from build123d import *

# Parameters (mm, degrees)
BOSS_EXTRUDE1_DEPTH = 3.175
CAVITY1_DEPTH       = 3.175


# Read off the part's stored shape, not the designer's step: Cavity1
with BuildPart() as part:
    # Sketch1 → Boss-Extrude1 (new body)
    with BuildSketch(Plane.XY):
        with BuildLine():
            Line((-9.017779189, 0), (0, 0))
            Line((0, 0), (0, 1.852083291))
            ThreePointArc((0, 1.852083291), (-2.38125, 4.233333291), (0, 6.614583291))
            Line((0, 6.614583291), (0, 20.902083291))
            ThreePointArc((0, 20.902083291), (-2.38125, 23.283333291), (0, 25.664583291))
            Line((0, 25.664583291), (0, 27.516666667))
            Line((0, 27.516666667), (-7.878035599, 27.516666667))
            ThreePointArc((-7.878035599, 27.516666667), (-12.19254052, 25.825802562), (-14.209331582, 21.653689435))
            Line((-14.209331582, 21.653689435), (-15.349075172, 6.837022768))
            ThreePointArc((-15.349075172, 6.837022768), (-13.676915084, 2.035495079), (-9.017779189, 0))
        make_face()
        with BuildLine():
            Line((0, 1.852083291), (0, 0))
            Line((0, 0), (9.017779189, 0))
            ThreePointArc((9.017779189, 0), (13.676915084, 2.035495079), (15.349075172, 6.837022768))
            Line((15.349075172, 6.837022768), (14.209331582, 21.653689435))
            ThreePointArc((14.209331582, 21.653689435), (12.19254052, 25.825802562), (7.878035599, 27.516666667))
            Line((7.878035599, 27.516666667), (0, 27.516666667))
            Line((0, 27.516666667), (0, 25.664583291))
            ThreePointArc((0, 25.664583291), (1.683798023, 24.967131314), (2.38125, 23.283333291))
            ThreePointArc((2.38125, 23.283333291), (1.683798023, 21.599535268), (0, 20.902083291))
            Line((0, 20.902083291), (0, 6.614583291))
            ThreePointArc((0, 6.614583291), (1.683798023, 5.917131314), (2.38125, 4.233333291))
            ThreePointArc((2.38125, 4.233333291), (1.683798023, 2.549535268), (0, 1.852083291))
        make_face()
    extrude(amount=BOSS_EXTRUDE1_DEPTH)

    # Cavity1 outline → Cavity1 (cut)
    with BuildSketch(Plane.XY):
        Polygon((11.287194974, 18.244530059), (11.939915796, 9.759159375), (15.105563788, 10.002670759), (14.452842966, 18.488041443), align=None)
        Polygon((-15.105563788, 10.002670759), (-11.939915796, 9.759159375), (-11.287194974, 18.244530059), (-14.452842966, 18.488041443), align=None)
    extrude(amount=CAVITY1_DEPTH, mode=Mode.SUBTRACT)


solid = part.part
The listing builds one solid part. Answer for the finished solid, in the listing's coordinates (mm). A direction names the side the tool comes from. Round coordinates to 2 decimals unless told otherwise and drop trailing zeros. Order: outer loops, then holes, each group sorted by start corner. A loop starts at its lowest first (then second) coordinate and runs counter-clockwise, first axis right, second up. Notation, with made-up numbers: (84, 32) - (133, 32) arc R29 ccw to (133, 55) - close; hole circle Ø11 at (-25.75, 53.5). An arc over 180 degrees is marked (long way). Write item = value, one per line. Start each with the question number.
1) Section A-A, the plane z = 2.55 is taken. Write down the section's boundary in (x, y).
2) For faces 4 (the flat face through (12.892, 18.368, 1.565)), 5 (the flat face through (-12.848, 18.365, 1.565)), 6 (the flat face through (14.333, 20.049, 1.565)), 7 (the flat face through (13.5, 9.88, 1.57)), 8 (the flat face through (-14.33, 20.09, 1.57)), determine the directions among +Z, -Z, +X, -X, +Y, -Y from which every point of the face is accessible in a straight line to the end or side of a thin tool.
3) Given pin 1 (1.5 mm diameter, centred on y = 4, z = 1.5, fed in from -X), flat-ended and moving along its own axis, determine where the tip first touches the part or whether it passes through.
4) Straight lines are drawn through the part: L1, parallel to Y at x = 2, z = 0.3; L2, parallel to Y at x = -13.5, z = 1.45; L3, parallel to X at y = 24.25, z = 0.8. For each, find the intervals that lie inside material, in ascending order.
5) For a pull along Y with two mould halves and no side action, classify faces 1 (the flat face through (0, 14, 3.175)), 2 (the flat face through (0, 27.517, 2)), 3 (the flat face through (-11.62, 13.94, 1.57)) as released by +Y, released by -Y, zero draft, split by the parting line, or undercut.
6) Section B-B, the plane x = 2 is taken. Write down the section's boundary in (y, z) (3 decimals).
Results list:
q1.outline = (-15.35, 6.84) arc R6.35 ccw to (-9.02, 0) - (9.02, 0) arc R6.35 ccw to (15.35, 6.84) - (15.11, 10) - (11.94, 9.76) - (11.29, 18.24) - (14.45, 18.49) - (14.21, 21.65) arc R6.35 ccw to (7.88, 27.52) - (-7.88, 27.52) arc R6.35 ccw to (-14.21, 21.65) - (-14.45, 18.49) - (-11.29, 18.24) - (-11.94, 9.76) - (-15.11, 10) - close; hole circle Ø4.76 at (0, 4.23); hole circle Ø4.76 at (0, 23.28)
q2.face_4 = +Z, -Z, +X
q2.face_5 = +Z, -Z, -X
q2.face_6 = +Z, -Z, +X, +Y
q2.face_7 = +Z, -Z
q2.face_8 = +Z, -Z, -X, +Y
q3.pin_1 = -15.16
q4.L1 = 0 to 2.94, 5.53 to 21.99, 24.58 to 27.52
q4.L2 = 1.85 to 9.88, 18.41 to 24.12
q4.L3 = -13.43 to -2.18, 2.18 to 13.43
q5.face_1 = zero draft
q5.face_2 = released by +Y
q5.face_3 = undercut
q6.outline = (0, 0) - (2.941, 0) - (2.941, 3.175) - (0, 3.175) - close; (5.526, 0) - (21.991, 0) - (21.991, 3.175) - (5.526, 3.175) - close; (24.576, 0) - (27.517, 0) - (27.517, 3.175) - (24.576, 3.175) - close
